```python
from build123d import *

# Parameters (mm, degrees)
SKETCH2_R           = 13.875
BOSS_EXTRUDE1_DEPTH = 8
BOSS_EXTRUDE2_DEPTH = 8
CIRPATTERN2_COUNT   = 21
SKETCH5_R           = 1.5
MIDDLE_HOLE_DEPTH   = 8


with BuildPart() as part:
    # Sketch2 → Boss-Extrude1 (new body)
    with BuildSketch(Plane.XY):
        Circle(SKETCH2_R)
    extrude(amount=BOSS_EXTRUDE1_DEPTH)

    # Sketch3 → Boss-Extrude2 (add)
    with BuildSketch(Plane.XY):
        with BuildLine():
            Line((0, 0), (1.325926716, 14.740485689))
            ThreePointArc((1.325926716, 14.740485689), (1.091950654, 16.044411319), (0.525585636, 17.241991177))
            Line((0.525585636, 17.241991177), (-0.525585636, 17.241991177))
            ThreePointArc((-0.525585636, 17.241991177), (-1.091950654, 16.044411319), (-1.325926716, 14.740485689))
            Line((-1.325926716, 14.740485689), (0, 0))
        make_face()
    boss_extrude2 = extrude(amount=BOSS_EXTRUDE2_DEPTH)

    # CirPattern2: Boss-Extrude2 ×21 about axis
    cirpattern2_axis = Axis((0, 0, 0), (0, 0, 1))
    for i in range(1, CIRPATTERN2_COUNT):
        add(boss_extrude2.rotate(cirpattern2_axis, i * 360 / CIRPATTERN2_COUNT))

    # Sketch5 → Middle Hole (cut)
    with BuildSketch(Plane.XY.offset(8)):
        Circle(SKETCH5_R)
    extrude(amount=-MIDDLE_HOLE_DEPTH, mode=Mode.SUBTRACT)


solid = part.part
```
Could you check a few things on this model? Use its own coordinates, in mm. A direction names the side the tool comes from. Coordinates: 2 decimals unless noted, no trailing zeros. Write each loop counter-clockwise with the first axis right and the second up, starting at its lowest first coordinate (ties: lowest second). Pieces come first, ordered by that corner, then holes. Notation, with made-up numbers: M 18,0 L 32,0 A11 cw 32,14 Z; hole C 7,1 d10. An arc over 180 degrees is marked long. Answer as CSV lines item,"result". Start each with the question number.
1) For faces 4 (the flat face through (-6.98, 12.52, 3.94)), 5 (the cylindrical face through (-9.43, 10.18, 3.94)), 6 (the cylindrical face through (-5.99, -14.94, 3.94)), 7 (the cylindrical face through (-15.35, 4.86, 3.94)), which set-ups out of +Z, -Z, +X, -X, +Y, -Y let a thin tool reach every point of the face, with its end or its side?
2) I want a section at B-B, the plane y = -10.5. Please give me the cut outline in (x, z).
3) I want a section at C-C, the plane y = 3. Please give me the cut outline in (x, z), and give its area (3 significant figures).
4) For P1, Ø4, axis at x = 8, z = 1, coming from the -Y side; P2, Ø1.5, axis at x = -7, z = 2, coming from the +Y side; P3, Ø3, axis at y = 14, z = 7, coming from the +X side, each with a flat end and sliding along its axis, tell me the tip position at first contact or that it passes through.
5) We'd pull the mould along Y, two halves only. Please class faces 1 (the flat face through (2.56, -17.05, 3.94)), 2 (the flat face through (-5.075, 16.478, 3.944)), 3 (the cylindrical face through (-15.418, -4.633, 3.944)): +Y half, -Y half, draft (parallel to the pull), parting line (faces both ways), or undercut.
6) Please list where these lines run through material, in increasing order: line 1 (Y direction, x = 0, z = 2) (3 decimals); line 2 (Y direction, x = 15, z = 7); line 3 (X direction, y = 13, z = 0.75). Write a range as from..to.
7) I want a section at A-A, the plane x = 0. Please give me the cut outline in (y, z) (3 decimals), and give its area (3 significant figures).
Data:
1,face 4,"+Z, -Z, +Y"
1,face 5,"+Z, -Z"
1,face 6,"+Z, -Z, -Y"
1,face 7,"+Z, -Z, -X"
2,outline,"M -11.43,0 L 11.43,0 L 11.43,8 L -11.43,8 Z"
3,outline,"M -13.55,0 L 13.55,0 L 13.55,8 L -13.55,8 Z"
3,area,"217 mm^2"
4,P1,"stops at y = -15.76"
4,P2,"stops at y = 13.54"
4,P3,"stops at x = 10.15"
5,face 1,"-Y half"
5,face 2,"+Y half"
5,face 3,"undercut"
6,line 1,"y = -13.875..-1.5, 1.5..17.242"
6,line 2,"y = -8.5..-7.82, -4.65..-2.09, -0.19..2.42, 4.6..6.89"
6,line 3,"x = -10.03..-7.26, -5.33..5.33, 7.26..10.03"
7,outline,"M -13.875,0 L -1.5,0 L -1.5,8 L -13.875,8 Z; M 1.5,0 L 17.242,0 L 17.242,8 L 1.5,8 Z"
7,area,"225 mm^2"
